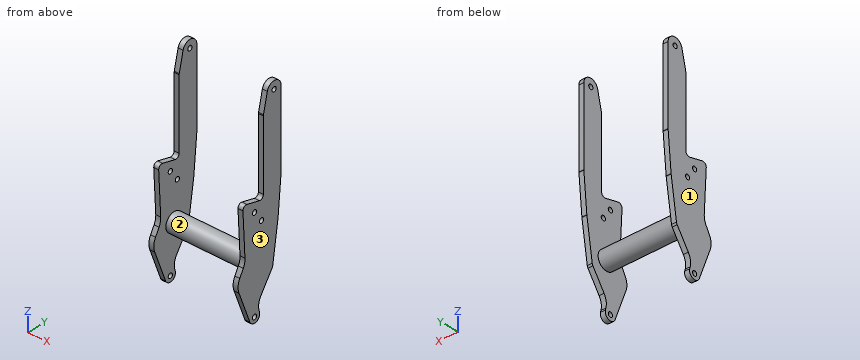
```python
from build123d import *

# Parameters (mm, degrees)
SKETCH1_R           = 4.75
BOSS_EXTRUDE1_DEPTH = 90
FILLET1_R           = 10
SKETCH4_W           = 160
SKETCH4_H           = 412.025
CUT_EXTRUDE2_DEPTH  = 418.739316622
SKETCH5_R           = 18.75
BOSS_EXTRUDE3_DEPTH = 90


with BuildPart() as part:
    # Sketch1 → Boss-Extrude1 (new, symmetric)
    with BuildSketch(Plane(origin=(0, 0, 0), x_dir=(0, 0, -1), z_dir=(1, 0, 0))):
        with BuildLine():
            Line((0, 15.625), (155.5, 15.625))
            Line((155.5, 15.625), (232.5, 8.888372909))
            Line((232.5, 8.888372909), (315, -3.441334703))
            Line((315, -3.441334703), (353.780445284, -29.599075334))
            ThreePointArc((353.780445284, -29.599075334), (365.491486019, -34.297330028), (378.098548324, -33.764364436))
            Line((378.098548324, -33.764364436), (382.133919944, -32.716161814))
            ThreePointArc((382.133919944, -32.716161814), (395.855263955, -40.268155018), (389.086597054, -54.392355215))
            Line((389.086597054, -54.392355215), (325.840301311, -78.678532537))
            ThreePointArc((325.840301311, -78.678532537), (312.996785566, -80.599492359), (300.544774533, -76.912568905))
            Line((300.544774533, -76.912568905), (286.274266107, -69.004404506))
            ThreePointArc((286.274266107, -69.004404506), (278.478171078, -66.012774583), (270.159478586, -65.285930348))
            Line((270.159478586, -65.285930348), (183.644750078, -69.829776728))
            ThreePointArc((183.644750078, -69.829776728), (177.69334539, -67.229235713), (176.212855636, -60.905456668))
            Line((176.212855636, -60.905456668), (182.866024409, -33.050687222))
            ThreePointArc((182.866024409, -33.050687222), (181.505326746, -26.874655225), (175.81438365, -24.116388374))
            Line((175.81438365, -24.116388374), (35, -24.116388374))
            Line((35, -24.116388374), (-3.514860224, -15.224532262))
            ThreePointArc((-3.514860224, -15.224532262), (-15.524560245, 1.768800215), (0, 15.625))
        make_face()
        with Locations(Location((0, 0, 0), (0, 0, 180))):
            Circle(SKETCH1_R, mode=Mode.SUBTRACT)
        with Locations(Location((198.75, -43.75, 0), (0, 0, 180))):
            Circle(SKETCH1_R, mode=Mode.SUBTRACT)
        with Locations(Location((220.5, -28, 0), (0, 0, 180))):
            Circle(SKETCH1_R, mode=Mode.SUBTRACT)
        with Locations(Location((385, -43.75, 0), (0, 0, 180))):
            Circle(SKETCH1_R, mode=Mode.SUBTRACT)
    extrude(amount=BOSS_EXTRUDE1_DEPTH, both=True)

    # Fillet1
    # the kernel refuses this fillet: 10 mm, written as the material it takes off along each edge
    with BuildSketch(Plane(origin=(91.091523573, 15.625, -155.5), x_dir=(0, 0, 1), z_dir=(-1, 0, 0))) as fillet1_piece_1:
        with BuildLine():
            CenterArc((FILLET1_R * 0.0436609429085, -FILLET1_R), FILLET1_R, 90, 5)
            Line((-FILLET1_R * 0.0434947998391, -FILLET1_R * 0.00380530190825), (0, 0))
            Line((0, 0), (FILLET1_R * 0.0436609429085, 0))
        make_face()
    extrude(amount=182.183047145, mode=Mode.SUBTRACT)
    with BuildSketch(Plane(origin=(90.763819082, 8.888372909, -232.5), x_dir=(0, -0.14780941112960186, -0.989015863361918), z_dir=(-1, 0, 0))) as fillet1_piece_2:
        with BuildLine():
            CenterArc((FILLET1_R * 0.0305527632986, FILLET1_R), FILLET1_R, 266.5, 3.5)
            Line((-FILLET1_R * 0.0304957762363, FILLET1_R * 0.00186520157813), (0, 0))
            Line((0, 0), (FILLET1_R * 0.0305527632986, 0))
        make_face()
    extrude(amount=181.527638165, mode=Mode.SUBTRACT)
    with BuildSketch(Plane(origin=(95.656922456, -3.441334703, -315), x_dir=(0, -0.5591929034707496, -0.8290375725550397), z_dir=(-1, 0, 0))) as fillet1_piece_3:
        with BuildLine():
            CenterArc((FILLET1_R * 0.226276898255, FILLET1_R), FILLET1_R, 244.5, 25.5)
            Line((-FILLET1_R * 0.204234198553, FILLET1_R * 0.0974147156501), (0, 0))
            Line((0, 0), (FILLET1_R * 0.226276898255, 0))
        make_face()
    extrude(amount=191.313844913, mode=Mode.SUBTRACT)
    with BuildSketch(Plane(origin=(-92.848390208, -24.116388374, -35), x_dir=(0, 0.2249510543438657, 0.9743700647852351), z_dir=(1, 0, 0))) as fillet1_piece_4:
        with BuildLine():
            CenterArc((FILLET1_R * 0.113935608302, -FILLET1_R), FILLET1_R, 90, 13)
            Line((-FILLET1_R * 0.111015446042, -FILLET1_R * 0.0256299352148), (0, 0))
            Line((0, 0), (FILLET1_R * 0.113935608302, 0))
        make_face()
    extrude(amount=185.696780415, mode=Mode.SUBTRACT)

    # Sketch4 → Cut-Extrude2 (cut, through all)
    with BuildSketch(Plane(origin=(0, 15.625, 0), x_dir=(1, 0, 0), z_dir=(0, 1, 0))):
        with Locations((0, 190.3875)):
            Rectangle(SKETCH4_W, SKETCH4_H)
    extrude(amount=-CUT_EXTRUDE2_DEPTH, mode=Mode.SUBTRACT)


with BuildPart() as cut_extrude2_piece_1:
    # of the separate pieces the step leaves, piece 1, a body of its own (cut_extrude2_pieces)
    add(part.part.solids().sort_by_distance((80, 15.625, 0))[0])



with BuildPart() as cut_extrude2_piece_2:
    # of the separate pieces the step leaves, piece 2, a body of its own (cut_extrude2_pieces)
    add(part.part.solids().sort_by_distance((-90, 15.625, 0))[0])


with BuildPart() as cut_extrude2_piece_1_1:
    add(cut_extrude2_piece_1.part)

    add(cut_extrude2_piece_2.part)  # Boss-Extrude3 merges Cut-Extrude2 piece 2
    # Sketch5 → Boss-Extrude3 (add, symmetric)
    with BuildSketch(Plane(origin=(0, 0, 0), x_dir=(0, 0, -1), z_dir=(1, 0, 0))):
        with Locations(Location((293.25, -35, 0), (0, 0, 180))):
            Circle(SKETCH5_R)
    extrude(amount=BOSS_EXTRUDE3_DEPTH, both=True)


solid = cut_extrude2_piece_1_1.part
```
Geometry check sheet. Reference: the model listing, model coordinates, mm. Face numbers are marked on the shaded views. Give positions to 0.01 mm unless a question says otherwise; leave off trailing zeros. Loops run counter-clockwise (first coordinate to the right, second up) from the corner with the lowest first, then second, coordinate; pieces in that order, holes last. Notation, with made-up numbers: M 82,20 L 118,20 A17 ccw 118,26 Z; hole C 41.5,56 d3. An arc over 180 degrees is marked long. Write item = value, one per line.
(1) Gauge pin test, flat ends, axial feed: pin 1 Ø7.5 at (y, z) = (-43.75, -198.75) entering from +X; pin 2 Ø8 at (x, z) = (85, -74) entering from -Y; pin 3 Ø8 at (x, y) = (-71, -32.5) entering from +Z; pin 4 Ø4 at (x, y) = (0.5, -41.5) entering from -Z. Record the tip position at first contact, or that the pin passes through.
Answer below:
pin_1 = through
pin_2 = -24.12
pin_3 = -274.5
pin_4 = -311.45
(2) Sectioned sample at D-D, the plane z = -293.25. Record the cut outline in (x, y).
Answer below:
outline = M -90,-72.87 L -80,-72.87 L -80,-53.75 L 80,-53.75 L 80,-72.87 L 90,-72.87 L 90,-0.19 L 80,-0.19 L 80,-16.25 L -80,-16.25 L -80,-0.19 L -90,-0.19 Z
(3) Material ranges on line 1 (X direction, y = -46.5, z = -204); line 2 (Z direction, x = 83.5, y = -43.75); line 3 (Z direction, x = 88, y = -43), recorded low to high. Write a range as [from, to].
Answer below:
line_1 = [-90, -80], [80, 90]
line_2 = [-396.4, -389.75], [-380.25, -203.5], [-194, -180.31]
line_3 = [-396.38, -389.69], [-380.31, -203.44], [-194.06, -180.49]
(4) Sectioned sample at B-B, the plane y = -43.75. Record the cut outline in (x, z).
Answer below:
outline = M -90,-396.4 L -80,-396.4 L -80,-389.75 L -90,-389.75 Z; M -90,-380.25 L -80,-380.25 L -80,-309.83 L 80,-309.83 L 80,-380.25 L 90,-380.25 L 90,-203.5 L 80,-203.5 L 80,-276.67 L -80,-276.67 L -80,-203.5 L -90,-203.5 Z; M -90,-194 L -80,-194 L -80,-180.31 L -90,-180.31 Z; M 80,-396.4 L 90,-396.4 L 90,-389.75 L 80,-389.75 Z; M 80,-194 L 90,-194 L 90,-180.31 L 80,-180.31 Z
(5) Sectioned sample at C-C, the plane x = 52. Record the cut outline in (y, z), plus the area to 3 significant figures.
Answer below:
outline = C -35,-293.25 d37.5
area = 1,100 mm2
(6) Release check for a two-part mould opening along X. For the marked faces 1, 2 and 3 record: released by +X, released by -X, zero draft, split by the parting line, or undercut.
Answer below:
face_1 = released by -X
face_2 = undercut
face_3 = released by +X
(7) Sectioned sample at A-A, the plane z = -251. Record the cut outline in (x, y), plus the area to 3 significant figures.
Answer below:
outline = M -90,-66.29 L -80,-66.29 L -80,6.12 L -90,6.12 Z; M 80,-66.29 L 90,-66.29 L 90,6.12 L 80,6.12 Z
area = 1,450 mm2
